from build123d import *

# Parameters (mm, degrees)
SKETCH1_R          = 2.6
BASE_FLANGE1_DEPTH = 3
FILLET1_R          = 5
FILLET2_R          = 5


# Sheet-metal steps are written as plain solids
with BuildPart() as part:
    # Sketch1 → Base-Flange1 (new body)
    with BuildSketch(Plane(origin=(0, 0, 0), x_dir=(1, 0, 0), z_dir=(0, 1, 0))):
        Polygon((32, 50), (50, 50), (50, -50), (-50, -50), (-50, -32), (25, -32), (32, -25), align=None)
        with Locations(Location((41, -41, 0), (0, 0, 270))):
            Circle(SKETCH1_R, mode=Mode.SUBTRACT)
        with Locations(Location((23, -41, 0), (0, 0, 270))):
            Circle(SKETCH1_R, mode=Mode.SUBTRACT)
        with Locations(Location((5, -41, 0), (0, 0, 270))):
            Circle(SKETCH1_R, mode=Mode.SUBTRACT)
        with Locations(Location((-13, -41, 0), (0, 0, 270))):
            Circle(SKETCH1_R, mode=Mode.SUBTRACT)
        with Locations(Location((-31, -41, 0), (0, 0, 270))):
            Circle(SKETCH1_R, mode=Mode.SUBTRACT)
        with Locations(Location((41, -23, 0), (0, 0, 270))):
            Circle(SKETCH1_R, mode=Mode.SUBTRACT)
        with Locations(Location((41, -5, 0), (0, 0, 270))):
            Circle(SKETCH1_R, mode=Mode.SUBTRACT)
        with Locations(Location((41, 13, 0), (0, 0, 270))):
            Circle(SKETCH1_R, mode=Mode.SUBTRACT)
        with Locations(Location((41, 31, 0), (0, 0, 270))):
            Circle(SKETCH1_R, mode=Mode.SUBTRACT)
    extrude(amount=-BASE_FLANGE1_DEPTH)

    # Fillet1
    fillet1_edges = [part.edges().sort_by_distance(p)[0] for p in [
        (25, -1.5, 32),
        (32, -1.5, 25),
    ]]
    fillet(fillet1_edges, radius=FILLET1_R)

    # Fillet2
    fillet2_edges = [part.edges().sort_by_distance(p)[0] for p in [
        (50, -1.5, 50),
        (-50, -1.5, 50),
        (-50, -1.5, 32),
        (32, -1.5, -50),
        (50, -1.5, -50),
    ]]
    fillet(fillet2_edges, radius=FILLET2_R)


solid = part.part
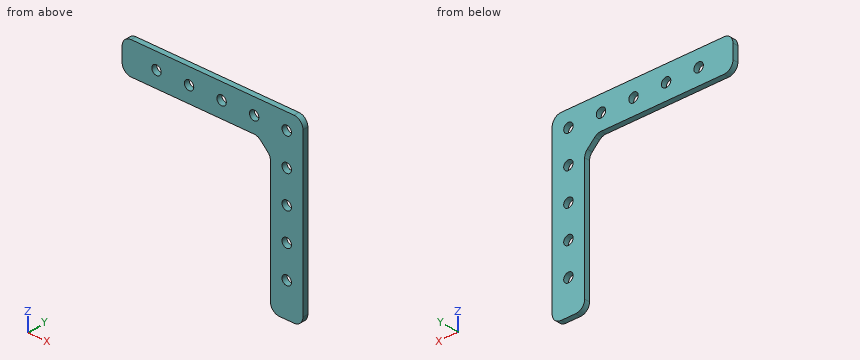
Work out the finished part from the listing and answer in its coordinate system (mm). Give positions to 0.01 mm unless a question says otherwise; leave off trailing zeros. Loops run counter-clockwise (first coordinate to the right, second up) from the corner with the lowest first, then second, coordinate; pieces in that order, holes last. Notation, with made-up numbers: (-22.75, 24.25) -> (6.25, 24.25) arc R16 ccw to (6.25, 50.25) -> close; hole circle Ø2 at (-17.5, 13.5). An arc over 180 degrees is marked (long way). Use a Markdown table: item, result. Add a question column.
1) The part is cut by section C-C, the plane y = -2.3. Count the separate pieces of the cut face and the enclosed holes in it, plus the area to 3 significant figures.
2) The part is cut by section B-B, the plane z = 6. Determine the outline of the cut face in (x, y), plus the area to 3 significant figures.
3) Consider line 1 along X through (y, z) = (-1.3, 41); line 2 along X through (y, z) = (-1.6, 23); line 3 along Z through (x, y) = (10.5, -0.3). Determine where each line is inside the solid, lowest interval first.
4) The part is cut by section D-D, the plane x = 41. Determine the outline of the cut face in (y, z), plus the area to 3 significant figures.
5) The part is cut by section A-A, the plane x = -13. Determine the outline of the cut face in (y, z).
6) This flat-tipped pin is pushed along its axis until it touches: P1, Ø0.9, axis at y = -1, z = -26, coming from the -X side. Where does it stop, or does it pass through?
Reported:
| question | item | result |
|---|---|---|
| 1 | separate pieces | 1 |
| 1 | enclosed holes | 9 |
| 1 | area | 3,080 mm^2 |
| 2 | outline | (32, -3) -> (38.6, -3) -> (38.6, 0) -> (32, 0) -> close; (43.4, -3) -> (50, -3) -> (50, 0) -> (43.4, 0) -> close |
| 2 | area | 39.6 mm^2 |
| 3 | line 1 | x = -50 to -33.6, -28.4 to -15.6, -10.4 to 2.4, 7.6 to 20.4, 25.6 to 38.4, 43.6 to 50 |
| 3 | line 2 | x = 32 to 38.4, 43.6 to 50 |
| 3 | line 3 | z = 32 to 50 |
| 4 | outline | (-3, -50) -> (0, -50) -> (0, -33.6) -> (-3, -33.6) -> close; (-3, -28.4) -> (0, -28.4) -> (0, -15.6) -> (-3, -15.6) -> close; (-3, -10.4) -> (0, -10.4) -> (0, 2.4) -> (-3, 2.4) -> close; (-3, 7.6) -> (0, 7.6) -> (0, 20.4) -> (-3, 20.4) -> close; (-3, 25.6) -> (0, 25.6) -> (0, 38.4) -> (-3, 38.4) -> close; (-3, 43.6) -> (0, 43.6) -> (0, 50) -> (-3, 50) -> close |
| 4 | area | 222 mm^2 |
| 5 | outline | (-3, 32) -> (0, 32) -> (0, 38.4) -> (-3, 38.4) -> close; (-3, 43.6) -> (0, 43.6) -> (0, 50) -> (-3, 50) -> close |
| 6 | P1 | stops at x = 32 |
